from build123d import *

# Parameters (mm, degrees)
SKETCH1_W           = 110
SKETCH1_H           = 100
SKETCH1_W_2         = 3
SKETCH1_H_2         = 3
BOSS_EXTRUDE1_DEPTH = 2.5
SKETCH2_W           = 110
SKETCH2_H           = 100
SKETCH2_W_2         = 20
SKETCH2_H_2         = 20
BOSS_EXTRUDE2_DEPTH = 2.5
SKETCH3_R           = 2.25
CUT_EXTRUDE1_DEPTH  = 6
CUT_EXTRUDE1_TAPER  = -8
SKETCH4_W           = 3
SKETCH4_H           = 3
CUT_EXTRUDE2_DEPTH  = 6.0000001
SKETCH5_W           = 10
SKETCH5_H           = 5
BOSS_EXTRUDE3_DEPTH = 20
SKETCH8_R           = 2.5
CUT_EXTRUDE4_DEPTH  = 15
SKETCH9_W           = 5
SKETCH9_H           = 10
BOSS_EXTRUDE4_DEPTH = 15
SKETCH10_R          = 2.5
CUT_EXTRUDE5_DEPTH  = 15


with BuildPart() as part:
    # Sketch1 → Boss-Extrude1 (new body)
    with BuildSketch(Plane(origin=(0, 0, 0), x_dir=(1, 0, 0), z_dir=(0, 1, 0))):
        with Locations((-55, 50)):
            Rectangle(SKETCH1_W, SKETCH1_H)
        with Locations((-59, 43.5)):
            Rectangle(SKETCH1_W_2, SKETCH1_H_2, mode=Mode.SUBTRACT)
        with Locations((-51, 43.5)):
            Rectangle(SKETCH1_W_2, SKETCH1_H_2, mode=Mode.SUBTRACT)
        with Locations((-55, 56.5)):
            Rectangle(SKETCH1_W_2, SKETCH1_H_2, mode=Mode.SUBTRACT)
    extrude(amount=BOSS_EXTRUDE1_DEPTH)

    # Sketch2 → Boss-Extrude2 (add)
    with BuildSketch(Plane(origin=(0, 2.5, 0), x_dir=(1, 0, 0), z_dir=(0, 1, 0))):
        with Locations((-55, 50)):
            Rectangle(SKETCH2_W, SKETCH2_H)
        with Locations((-55, 50)):
            Rectangle(SKETCH2_W_2, SKETCH2_H_2, mode=Mode.SUBTRACT)
    extrude(amount=BOSS_EXTRUDE2_DEPTH)

    # Sketch3 → Cut-Extrude1 (cut, through all)
    with BuildSketch(Plane(origin=(0, 5, 0), x_dir=(1, 0, 0), z_dir=(0, 1, 0))):
        with Locations((-82.921200256, 74.97538555)):
            Circle(SKETCH3_R)
    extrude(amount=-CUT_EXTRUDE1_DEPTH, taper=CUT_EXTRUDE1_TAPER, mode=Mode.SUBTRACT)

    # Sketch4 → Cut-Extrude2 (cut, through all)
    with BuildSketch(Plane(origin=(0, 5, 0), x_dir=(1, 0, 0), z_dir=(0, 1, 0))):
        with Locations((-22.5, 24.5)):
            Rectangle(SKETCH4_W, SKETCH4_H)
        with Locations((-16.5, 24.5)):
            Rectangle(SKETCH4_W, SKETCH4_H)
        with Locations((-22.5, 16.5)):
            Rectangle(SKETCH4_W, SKETCH4_H)
        with Locations((-16.5, 16.5)):
            Rectangle(SKETCH4_W, SKETCH4_H)
    extrude(amount=-CUT_EXTRUDE2_DEPTH, mode=Mode.SUBTRACT)

    # Sketch5 → Boss-Extrude3 (add)
    with BuildSketch(Plane(origin=(0, 5, 0), x_dir=(1, 0, 0), z_dir=(0, 1, 0))):
        with Locations((-15, 87.5)):
            Rectangle(SKETCH5_W, SKETCH5_H)
    extrude(amount=-BOSS_EXTRUDE3_DEPTH)

    # Sketch8 → Cut-Extrude4 (cut)
    with BuildSketch(Plane(origin=(0, 0, -90), x_dir=(-1, 0, 0), z_dir=(0, 0, -1))):
        with Locations((15, -10)):
            Circle(SKETCH8_R)
    extrude(amount=-CUT_EXTRUDE4_DEPTH, mode=Mode.SUBTRACT)

    # Sketch9 → Boss-Extrude4 (add)
    with BuildSketch(Plane.XZ):
        with Locations((-102.5, -10)):
            Rectangle(SKETCH9_W, SKETCH9_H)
    extrude(amount=BOSS_EXTRUDE4_DEPTH)

    # Sketch10 → Cut-Extrude5 (cut)
    with BuildSketch(Plane.ZY.offset(105)):
        with Locations((-10, -10)):
            Circle(SKETCH10_R)
    extrude(amount=-CUT_EXTRUDE5_DEPTH, mode=Mode.SUBTRACT)


solid = part.part
Build history of the part. All positions in model axes, mm. A direction names the side the tool comes from. Coordinates: 2 decimals unless noted, no trailing zeros. Order: outer loops, then holes, each group sorted by start corner. A loop starts at its lowest first (then second) coordinate and runs counter-clockwise, first axis right, second up. Notation, with made-up numbers: (22, 39.5) - (79, 39.5) arc R14 ccw to (79, 50.5) - close; hole circle Ø9 at (-29.5, -1). An arc over 180 degrees is marked (long way). Write each question's results on one line, items separated by ' | '. Start each with the question number.
Item 1: Band-saw the part on C-C on y = -10. Write the cut outline in (x, z), and give its area (3 significant figures).
Item 2: Tool access for faces 4 (the face through (-103, -7, -5)), 5 (the face through (-59, 1, -42)), 6 (the face through (-103, -7, -15)), 7 (the face through (-103, -15, -10)): list every direction of +Z, -Z, +X, -X, +Y, -Y with a clear straight run to the whole face (end or side of a thin tool).
Item 3: Band-saw the part on A-A on z = -10. Write the cut outline in (x, y), and give its area (3 significant figures).
Item 4: Band-saw the part on B-B on y = -4. Write the cut outline in (x, z).
Item 5: Mould opens along X. For faces 1 (the face through (-56, 0, -51)), 2 (the face through (-45, 4, -50)), 3 (the face through (-100, -7, -10)) say: released by +X, released by -X, zero draft, split by the parting line, or undercut.
Item 6: Flat gauge pins, fed straight in: pin 1 (4 mm diameter, centred on x = -95, z = -90, fed in from -Y); pin 2 (5 mm diameter, centred on y = -10, z = -11.5, fed in from -X); pin 3 (5 mm diameter, centred on y = -7.5, z = -8.5, fed in from +X). Where does each tip first touch, or does it go through?
Item 7: Wall check: probe 1 along Y at (x, z) = (-15, -88); probe 2 along Z at (x, y) = (-55, 0.75); probe 3 along Y at (x, z) = (-77.5, -24). Give the ranges that are in metal, low to high. Write a range as [from, to].
Item 8: Band-saw the part on D-D on x = -35. Write the cut outline in (y, z).
Numbers:
1) outline: (-105, -15) - (-100, -15) - (-100, -12.5) - (-105, -12.5) - close; (-105, -7.5) - (-100, -7.5) - (-100, -5) - (-105, -5) - close; (-20, -90) - (-17.5, -90) - (-17.5, -85) - (-20, -85) - close; (-12.5, -90) - (-10, -90) - (-10, -85) - (-12.5, -85) - close | area: 50.0 mm^2
2) face 4: +Z, +X, -X, -Y | face 5: +Y, -Y | face 6: -Z, +X, -X, -Y | face 7: +Z, -Z, +X, -X, -Y
3) outline: (-110, 0) - (-105, 0) - (-105, -7.5) - (-100, -7.5) - (-100, 0) - (0, 0) - (0, 5) - (-110, 5) - close; (-105, -15) - (-100, -15) - (-100, -12.5) - (-105, -12.5) - close | area: 600 mm^2
4) outline: (-105, -15) - (-100, -15) - (-100, -5) - (-105, -5) - close; (-20, -90) - (-10, -90) - (-10, -85) - (-20, -85) - close
5) face 1: zero draft | face 2: undercut | face 3: released by +X
6) pin 1: y = 0 | pin 2: x = -105 | pin 3: x = -100
7) probe 1: [-15, -12.5], [-7.5, 5] | probe 2: [-100, -58], [-55, 0] | probe 3: [0, 5]
8) outline: (0, -100) - (5, -100) - (5, 0) - (0, 0) - close
